from build123d import *

# Parameters (mm, degrees)
F1_DEPTH = 7.9375
F2_R     = 3.96874
F3_R     = 2.54
F4_DEPTH = 11.90625


# Not quite as in the source:
# - a fillet or chamfer is up to 0.001 mm smaller than in the source, because OpenCascade refuses the exact size


with BuildPart() as f1:
    # F0 (on Top) → F1 (new body)
    with BuildSketch(Plane.XY):
        Polygon((45.24375, 0), (0, 0), (0, -7.9375), (41.9559298487, -7.9375), (45.9246798487, -11.90625), (58.7375, -11.90625), (58.7375, -3.96875), (49.2125, -3.96875), align=None)
    extrude(amount=F1_DEPTH)

    # F2 (radius 3.96875 in the source; OpenCascade refuses exactly that, so slightly less here)
    f2_edges = [f1.edges().sort_by_distance(p)[0] for p in [
        (0, -3.96875, 0),
        (0, -3.96875, 7.9375),
        (58.7375, -7.9375, 0),
        (58.7375, -7.9375, 7.9375),
    ]]
    fillet(f2_edges, radius=F2_R)

    # F3 (on face) → F4 (cut, through all)
    with BuildSketch(Plane(origin=(0, 0, 0), x_dir=(-1, 0, 0), z_dir=(0, 1, 0))):
        with Locations((-3.96875, 3.96875)):
            Circle(F3_R)
        with Locations((-54.76875, 3.96875)):
            Circle(F3_R)
    extrude(amount=-F4_DEPTH, mode=Mode.SUBTRACT)


solid = f1.part
Geometry: final body of the model. Coordinates: model frame, mm. A direction names the side the tool comes from. Coordinates: 2 decimals unless noted, no trailing zeros. Loops run counter-clockwise (first coordinate to the right, second up) from the corner with the lowest first, then second, coordinate; pieces in that order, holes last. Notation, with made-up numbers: M 27.5,-24 L 47.5,-24 A16 cw 47.5,4 Z; hole C 3,-13.5 d8. An arc over 180 degrees is marked long. One line per item, written item: value. Start each with the question number.
1) Reachability of faces 5 (the flat face through (51, -11.906, 4)), 6 (the flat face through (21, -7.938, 4)) from +Z, -Z, +X, -X, +Y, -Y: full face, straight path, thin tool, end or side. Return the list, or none.
2) Cut plane A-A (y = -4.75). Count the separate pieces of the cut face and the enclosed holes in it, then the cut area to 3 significant figures.
3) Draft query along X for faces 1 (the cylindrical face through (4.299, -3.913, 6.487)), 2 (the cylindrical face through (52.346, -7.882, 4.732)), 3 (the flat face through (52, -3.969, 4)), 4 (the cylindrical face through (1.132, -4.024, 1.193)). Return one class per face: released by +X, released by -X, zero draft, split by the parting line, or undercut.
4) Pin query (flat end, axial travel): P1, Ø1.5, axis at y = -3.5, z = 6, coming from the -X side; P2, Ø2.5, axis at x = 55.5, z = 5.5, coming from the +Y side. Return the tip coordinate at first contact, or that it passes through.
5) Cut plane D-D (x = 13). Return loops of the section in (y, z).
6) Material intervals for L1, parallel to X at y = -7, z = 5.75; L2, parallel to Z at x = 4.5, y = -1.5; L3, parallel to Y at x = 10.5, z = 1.5, sorted ascending. Write a range as from..to.
7) Cut plane C-C (z = 5.5). Return loops of the section in (x, y), then the cut area to 3 significant figures.
Evaluation:
1. face 5: +Z, -Z, +X, -X, -Y
1. face 6: +Z, -Z, -X, -Y
2. separate pieces: 1
2. enclosed holes: 2
2. area: 412 mm^2
3. face 1: undercut
3. face 2: undercut
3. face 3: zero draft
3. face 4: released by -X
4. P1: x = 0.21
4. P2: y = -3.97
5. outline: M -7.94,0 L 0,0 L 0,7.94 L -7.94,7.94 Z
6. L1: 0.42..2.16, 5.78..52.96, 56.58..58.32
6. L2: 0..1.48, 6.45..7.94
6. L3: -7.94..0
7. outline: M 0.31,-7.94 L 1.94,-7.94 L 1.94,0 L 0.31,0 Z; M 6,-7.94 L 41.96,-7.94 L 45.92,-11.91 L 52.74,-11.91 L 52.74,-3.97 L 49.21,-3.97 L 45.24,0 L 6,0 Z; M 56.8,-11.91 L 58.43,-11.91 L 58.43,-3.97 L 56.8,-3.97 Z
7. area: 410 mm^2
